Here's how the part is built. I have some questions about the finished solid (model axes, mm). Face numbers are marked on the shaded views. A direction names the side the tool comes from. Give positions to 0.01 mm unless a question says otherwise; leave off trailing zeros. Loops run counter-clockwise (first coordinate to the right, second up) from the corner with the lowest first, then second, coordinate; pieces in that order, holes last. Notation, with made-up numbers: (27, 83.25) - (62, 83.25) arc R26 cw to (62, 113.25) - close; hole circle Ø6 at (-27.75, 43.25). An arc over 180 degrees is marked (long way). Put each result on its own line as item: value. Start each with the question number.
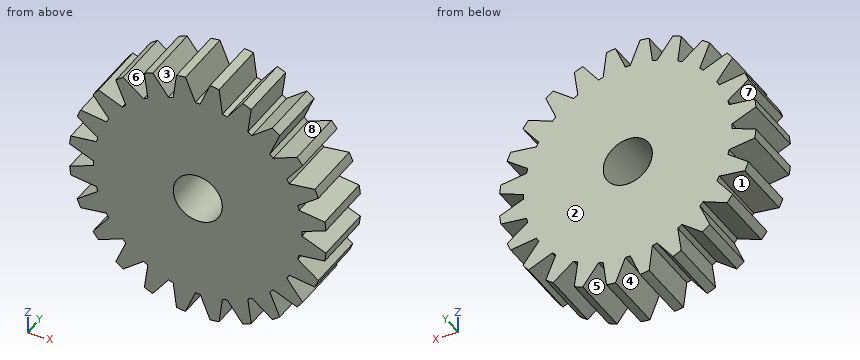
from build123d import *

# Parameters (mm, degrees)
SKETCH1_R           = 10.5
BOSS_EXTRUDE1_DEPTH = 5
SKETCH2_R           = 2
CUT_EXTRUDE1_DEPTH  = 6
CUT_EXTRUDE2_DEPTH  = 5
CIRPATTERN1_COUNT   = 24


with BuildPart() as part:
    # Sketch1 → Boss-Extrude1 (new body)
    with BuildSketch(Plane(origin=(0, 0, 0), x_dir=(1, 0, 0), z_dir=(0, 1, 0))):
        Circle(SKETCH1_R)
    extrude(amount=BOSS_EXTRUDE1_DEPTH)

    # Sketch2 → Cut-Extrude1 (cut, through all)
    with BuildSketch(Plane(origin=(0, 5, 0), x_dir=(1, 0, 0), z_dir=(0, 1, 0))):
        Circle(SKETCH2_R)
    extrude(amount=-CUT_EXTRUDE1_DEPTH, mode=Mode.SUBTRACT)

    # Sketch3 → Cut-Extrude2 (cut)
    with BuildSketch(Plane(origin=(0, 5, 0), x_dir=(1, 0, 0), z_dir=(0, 1, 0))):
        Polygon((0, 8.5), (0.2, 8.5), (1, 10.45227248), (1, 11.821377403), (-1, 11.821377403), (-1, 10.45227248), (-0.2, 8.5), align=None)
    cut_extrude2 = extrude(amount=-CUT_EXTRUDE2_DEPTH, mode=Mode.SUBTRACT)

    # CirPattern1: Cut-Extrude2 ×24 about axis
    cirpattern1_axis = Axis((0, 0, 0), (0, 1, 0))
    for i in range(1, CIRPATTERN1_COUNT):
        add(cut_extrude2.rotate(cirpattern1_axis, i * 360 / CIRPATTERN1_COUNT), mode=Mode.SUBTRACT)


solid = part.part
1) I'm going to push a flat-ended pin straight in: P1, Ø1.5, axis at x = 5.5, y = 1.5, coming from the -Z side. Where does the tip first touch, or does it pass through?
2) I need wall thicknesses on line 1 (Z direction, x = 0, y = 3.3); line 2 (Z direction, x = -9.25, y = 3.75). Which ranges of each line are inside material? Lowest first, please.
3) Which directions (+Z, -Z, +X, -X, +Y, -Y) give clear straight access to the entire face, cutting with the end or side of a thin tool? Please do the marked faces 5, 6, 7 and 8.
4) Suppose I cut it at A-A on x = 9.25. Please give me the cut outline in (y, z).
5) Suppose I cut it at B-B on x = 5. Please give me the cut outline in (y, z).
6) Thinking about a two-plate mould opening in Z: for the marked faces 1, 2, 3 and 4, which applies, pulls with the +Z half, pulls with the -Z half, needs draft (parallel to the pull), parting line crosses it, or undercut?
Ans:
1. P1: stops at z = -8.55
2. line 1: z = -8.5 to -2, 2 to 8.5
2. line 2: z = -4.32 to -3.22, -1.88 to -0.51, 0.51 to 1.88, 3.22 to 4.32
3. face 5: -Z, +Y, -Y
3. face 6: +Z, +Y, -Y
3. face 7: -X, +Y, -Y
3. face 8: +Y, -Y
4. outline: (0, -4.32) - (5, -4.32) - (5, -3.22) - (0, -3.22) - close; (0, -1.88) - (5, -1.88) - (5, -0.51) - (0, -0.51) - close; (0, 0.51) - (5, 0.51) - (5, 1.88) - (0, 1.88) - close; (0, 3.22) - (5, 3.22) - (5, 4.32) - (0, 4.32) - close
5. outline: (0, -7.71) - (5, -7.71) - (5, 7.71) - (0, 7.71) - close
6. face 1: undercut
6. face 2: needs draft
6. face 3: pulls with the +Z half
6. face 4: pulls with the -Z half
